Here's how the part is built. I have some questions about the finished solid (model axes, mm). A direction names the side the tool comes from. Coordinates: 2 decimals unless noted, no trailing zeros. Order: outer loops, then holes, each group sorted by start corner. A loop starts at its lowest first (then second) coordinate and runs counter-clockwise, first axis right, second up. Notation, with made-up numbers: (54.25, 7.5) - (61.25, 7.5) arc R15 cw to (61.25, 15.5) - close; hole circle Ø11 at (-23.75, -19.75). An arc over 180 degrees is marked (long way). Answer in a Markdown table with one row per item. Add a question column.
Item 1: I want a section at C-C (y = -51.5). Please give me the cut outline in (x, z) (3 decimals).
Item 2: If I drill on line 1 along Y through (x, z) = (0, -1.75); line 2 along Y through (x, z) = (0, 1.75) (3 decimals); line 3 along X through (y, z) = (-1, 3.75), over which ranges is the centre line in solid material (lowest first)? Write a range as from..to.
Item 3: On a 3-axis mill with a long thin cutter (end or side, diameter ignored), from which of +Z, -Z, +X, -X, +Y, -Y can I reach the whole of each face in a straight line? I mean faces 1 (the cylindrical face through (-0.879, 12.057, -2.007)), 2 (the cylindrical face through (18.63, -6.23, -1.49)), 3 (the flat face through (-15.599, -4.768, 1.021)). Say none if no direction works.
Item 4: Will these pins go through, and if not, where does the flat tip stop? pin 1 Ø0.8 at (y, z) = (-50.5, 3.5) entering from +X; pin 2 Ø0.8 at (x, z) = (48.5, 3) entering from +Y; pin 3 Ø0.9 at (y, z) = (-7.5, 1) entering from +X.
Item 5: I want a section at A-A (y = -8). Count the separate pieces of the cut face and the enclosed holes in it, plus the area to 3 significant figures.
```python
from build123d import *

# Parameters (mm, degrees)
F0_R              = 67
F1_DEPTH          = 2.5
F2_R              = 64.375
F2_R_2            = 62.625
F3_DEPTH          = 3
F2_R_3            = 58.875
F4_DEPTH          = 2
F5_R              = 4.75
F5_R_2            = 5.75
F5_R_3            = 2.1
F6_DEPTH          = 25
F7_R              = 5.75
F7_R_2            = 4.75
F8_DEPTH          = 0.5
F7_R_3            = 6.75
F9_DEPTH          = 1
F7_R_4            = 2.1
F10_DEPTH         = 3
F11_R             = 6.75
F11_R_2           = 5.75
F12_DEPTH         = 1
F13_W             = 5
F13_H             = 12
F14_DEPTH         = 1.5
F14_COPIES_COUNT  = 6
F14_COPIES_ANGLE  = 150
F14_COPIES1_COUNT = 6
F14_COPIES1_ANGLE = 150


# Not quite as in the source:
# - a feature of the source that left no trace in its solid (it failed there, or was rolled back) is left out
# - a pattern or mirror of a feature is missing from the dataset's text; its kind, count and spacing are read off the source's solid


with BuildPart() as f1:
    # F0 (on Top) → F1 (new body, symmetric)
    with BuildSketch(Plane.XY):
        Circle(F0_R)
    extrude(amount=F1_DEPTH, both=True)

    # F2 (on face) → F3 (join)
    with BuildSketch(Plane.XY.offset(2.5)):
        Circle(F2_R)
        Circle(F2_R_2, mode=Mode.SUBTRACT)
    extrude(amount=F3_DEPTH)

    # F2 (on face) → F4 (cut)
    with BuildSketch(Plane.XY.offset(2.5)):
        Circle(F2_R_2)
        Circle(F2_R_3, mode=Mode.SUBTRACT)
    extrude(amount=-F4_DEPTH, mode=Mode.SUBTRACT)

    # F5 (on face) → F6 (cut)
    with BuildSketch(Plane.XY.offset(2.5)):
        Circle(F5_R)
        with Locations((0, 18.75)):
            Circle(F5_R_2)
        with Locations((0, 46.25)):
            Circle(F5_R_2)
        with Locations((17.5, -8)):
            Circle(F5_R_3)
        with Locations((-17.5, -8)):
            Circle(F5_R_3)
    extrude(amount=-F6_DEPTH, mode=Mode.SUBTRACT)

    # F7 (on face) → F8 (cut)
    with BuildSketch(Plane.XY.offset(2.5)):
        Circle(F7_R)
        Circle(F7_R_2, mode=Mode.SUBTRACT)
    extrude(amount=-F8_DEPTH, mode=Mode.SUBTRACT)

    # F7 (on face) → F9 (cut)
    with BuildSketch(Plane.XY.offset(2.5)):
        with Locations((0, 18.75)):
            Circle(F7_R_3)
        with Locations((0, 18.75)):
            Circle(F7_R, mode=Mode.SUBTRACT)
        with Locations((0, 46.25)):
            Circle(F7_R_3)
        with Locations((0, 46.25)):
            Circle(F7_R, mode=Mode.SUBTRACT)
    extrude(amount=-F9_DEPTH, mode=Mode.SUBTRACT)

    # F7 (on face) → F10 (cut)
    with BuildSketch(Plane.XY.offset(2.5)):
        Polygon((-13.75, -10.1650635095), (-13.75, -5.8349364905), (-17.5, -3.6698729811), (-21.25, -5.8349364905), (-21.25, -10.1650635095), (-17.5, -12.3301270189), align=None)
        with Locations((-17.5, -8)):
            Circle(F7_R_4, mode=Mode.SUBTRACT)
        Polygon((21.25, -10.1650635095), (21.25, -5.8349364905), (17.5, -3.6698729811), (13.75, -5.8349364905), (13.75, -10.1650635095), (17.5, -12.3301270189), align=None)
        with Locations((17.5, -8)):
            Circle(F7_R_4, mode=Mode.SUBTRACT)
    extrude(amount=-F10_DEPTH, mode=Mode.SUBTRACT)

    # F11 (on face) → F12 (cut)
    with BuildSketch(Plane(origin=(0, 0, -2.5), x_dir=(1, 0, 0), z_dir=(0, 0, -1))):
        with Locations((0, -18.75)):
            Circle(F11_R)
        with Locations((0, -18.75)):
            Circle(F11_R_2, mode=Mode.SUBTRACT)
        with Locations((0, -46.25)):
            Circle(F11_R)
        with Locations((0, -46.25)):
            Circle(F11_R_2, mode=Mode.SUBTRACT)
    extrude(amount=-F12_DEPTH, mode=Mode.SUBTRACT)

    # F13 (on face) → F14 (join)
    with BuildSketch(Plane.XY.offset(2.5)):
        with Locations((0, -50)):
            Rectangle(F13_W, F13_H)
    f14 = extrude(amount=F14_DEPTH)

    # F14_copies: F14 ×6 about axis
    f14_copies_axis = Axis((0, 0, 0), (0, 0, 1))
    for i in range(1, F14_COPIES_COUNT):
        add(f14.rotate(f14_copies_axis, i * F14_COPIES_ANGLE / (F14_COPIES_COUNT - 1)))

    # F14_copies1: F14 ×6 about axis
    f14_copies1_axis = Axis((0, 0, 0), (0, 0, -1))
    for i in range(1, F14_COPIES1_COUNT):
        add(f14.rotate(f14_copies1_axis, i * F14_COPIES1_ANGLE / (F14_COPIES1_COUNT - 1)))


solid = f1.part
```
Values follow:
| question | item | result |
|---|---|---|
| 1 | outline | (-42.857, -2.5) - (42.857, -2.5) - (42.857, 2.5) - (38.625, 2.5) - (38.625, 5.5) - (35.632, 5.5) - (35.632, 0.5) - (28.531, 0.5) - (28.531, 2.5) - (2.5, 2.5) - (2.5, 4) - (-2.5, 4) - (-2.5, 2.5) - (-28.531, 2.5) - (-28.531, 0.5) - (-35.632, 0.5) - (-35.632, 5.5) - (-38.625, 5.5) - (-38.625, 2.5) - (-42.857, 2.5) - close |
| 2 | line 1 | y = -67..-4.75, 4.75..12, 25.5..39.5, 53..67 |
| 2 | line 2 | y = -67..-62.625, -58.875..-4.75, 4.75..12, 25.5..39.5, 53..58.875, 62.625..67 |
| 2 | line 3 | x = -64.37..-62.62, -56..-44, 44..56, 62.62..64.37 |
| 3 | face 1 | -Z |
| 3 | face 2 | +Z, -Z |
| 3 | face 3 | +Z |
| 4 | pin 1 | stops at x = 40.42 |
| 4 | pin 2 | stops at y = 42.78 |
| 4 | pin 3 | stops at x = 66.63 |
| 5 | separate pieces | 3 |
| 5 | enclosed holes | 0 |
| 5 | area | 599 mm^2 |
